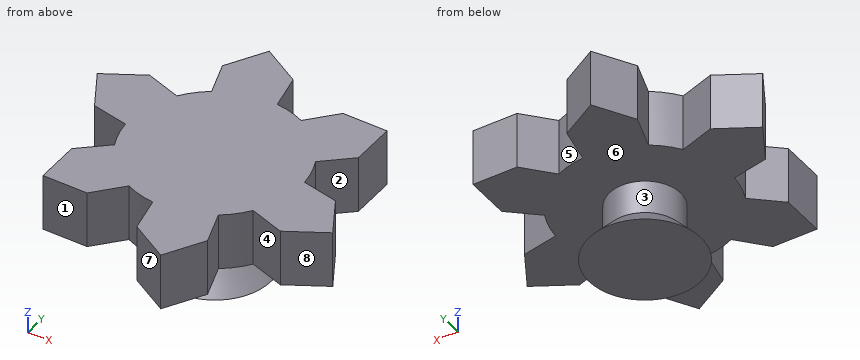
```python
from build123d import *

# Parameters (mm, degrees)
F1_DEPTH = 2.54
F2_R     = 1.5875
F3_DEPTH = 1.5
F4_R     = 2.5
F5_DEPTH = 1


with BuildPart() as f1:
    # F0 (on Top) → F1 (new body)
    with BuildSketch(Plane.XY):
        with BuildLine():
            ThreePointArc((1.6168332291, 3.4499203338), (1.7625208147, 3.3778129578), (1.905, 3.2995567884))
            ThreePointArc((1.905, 3.2995567884), (2.6940768363, 2.6940768363), (3.2995567884, 1.905))
            ThreePointArc((3.2995567884, 1.905), (3.3778129578, 1.7625208147), (3.4499203338, 1.6168332291))
            Line((3.4499203338, 1.6168332291), (4.669733183, 2.6960717102))
            Line((4.669733183, 2.6960717102), (4.669733183, 4.669733183))
            Line((4.669733183, 4.669733183), (2.6960717102, 4.669733183))
            Line((2.6960717102, 4.669733183), (1.6168332291, 3.4499203338))
        make_face()
        with BuildLine():
            Line((1.905, 3.2995567884), (0, 0))
            Line((0, 0), (3.2995567884, 1.905))
            ThreePointArc((3.2995567884, 1.905), (2.6940768363, 2.6940768363), (1.905, 3.2995567884))
        make_face()
        with BuildLine():
            ThreePointArc((0.3247415168, 3.7961352646), (0.1625186786, 3.806532238), (0, 3.81))
            Line((0, 3.81), (0, 0))
            Line((0, 0), (1.905, 3.2995567884))
            ThreePointArc((1.905, 3.2995567884), (1.7625208147, 3.3778129578), (1.6168332291, 3.4499203338))
            ThreePointArc((1.6168332291, 3.4499203338), (0.9861005618, 3.6801773982), (0.3247415168, 3.7961352646))
        make_face()
        with BuildLine():
            ThreePointArc((-1.905, 3.2995567884), (-0.9861005618, 3.6801773982), (0, 3.81))
            ThreePointArc((0, 3.81), (0.1625186786, 3.806532238), (0.3247415168, 3.7961352646))
            Line((0.3247415168, 3.7961352646), (0, 5.3921434204))
            Line((0, 5.3921434204), (-1.7092409739, 6.3789741568))
            Line((-1.7092409739, 6.3789741568), (-2.6960717102, 4.669733183))
            Line((-2.6960717102, 4.669733183), (-2.1793020355, 3.125178817))
            ThreePointArc((-2.1793020355, 3.125178817), (-2.0440114233, 3.2152942791), (-1.905, 3.2995567884))
        make_face()
        with BuildLine():
            Line((0, 0), (0, 3.81))
            ThreePointArc((0, 3.81), (-0.9861005618, 3.6801773982), (-1.905, 3.2995567884))
            Line((-1.905, 3.2995567884), (0, 0))
        make_face()
        with BuildLine():
            Line((-3.2995567884, 1.905), (0, 0))
            Line((0, 0), (-1.905, 3.2995567884))
            ThreePointArc((-1.905, 3.2995567884), (-2.0440114233, 3.2152942791), (-2.1793020355, 3.125178817))
            ThreePointArc((-2.1793020355, 3.125178817), (-2.6940768363, 2.6940768363), (-3.125178817, 2.1793020355))
            ThreePointArc((-3.125178817, 2.1793020355), (-3.2152942791, 2.0440114233), (-3.2995567884, 1.905))
        make_face()
        with BuildLine():
            ThreePointArc((-3.7961352646, -0.3247415168), (-3.806532238, -0.1625186786), (-3.81, 0))
            ThreePointArc((-3.81, 0), (-3.6801773982, 0.9861005618), (-3.2995567884, 1.905))
            ThreePointArc((-3.2995567884, 1.905), (-3.2152942791, 2.0440114233), (-3.125178817, 2.1793020355))
            Line((-3.125178817, 2.1793020355), (-4.669733183, 2.6960717102))
            Line((-4.669733183, 2.6960717102), (-6.3789741568, 1.7092409739))
            Line((-6.3789741568, 1.7092409739), (-5.3921434204, 0))
            Line((-5.3921434204, 0), (-3.7961352646, -0.3247415168))
        make_face()
        with BuildLine():
            Line((-3.81, 0), (0, 0))
            Line((0, 0), (-3.2995567884, 1.905))
            ThreePointArc((-3.2995567884, 1.905), (-3.6801773982, 0.9861005618), (-3.81, 0))
        make_face()
        with BuildLine():
            Line((-3.2995567884, -1.905), (0, 0))
            Line((0, 0), (-3.81, 0))
            ThreePointArc((-3.81, 0), (-3.806532238, -0.1625186786), (-3.7961352646, -0.3247415168))
            ThreePointArc((-3.7961352646, -0.3247415168), (-3.6801773982, -0.9861005618), (-3.4499203338, -1.6168332291))
            ThreePointArc((-3.4499203338, -1.6168332291), (-3.3778129578, -1.7625208147), (-3.2995567884, -1.905))
        make_face()
        with BuildLine():
            Line((-1.905, -3.2995567884), (0, 0))
            Line((0, 0), (-3.2995567884, -1.905))
            ThreePointArc((-3.2995567884, -1.905), (-2.6940768363, -2.6940768363), (-1.905, -3.2995567884))
        make_face()
        with BuildLine():
            ThreePointArc((-1.6168332291, -3.4499203338), (-1.7625208147, -3.3778129578), (-1.905, -3.2995567884))
            ThreePointArc((-1.905, -3.2995567884), (-2.6940768363, -2.6940768363), (-3.2995567884, -1.905))
            ThreePointArc((-3.2995567884, -1.905), (-3.3778129578, -1.7625208147), (-3.4499203338, -1.6168332291))
            Line((-3.4499203338, -1.6168332291), (-4.669733183, -2.6960717102))
            Line((-4.669733183, -2.6960717102), (-4.669733183, -4.669733183))
            Line((-4.669733183, -4.669733183), (-2.6960717102, -4.669733183))
            Line((-2.6960717102, -4.669733183), (-1.6168332291, -3.4499203338))
        make_face()
        with BuildLine():
            Line((0, -3.81), (0, 0))
            Line((0, 0), (-1.905, -3.2995567884))
            ThreePointArc((-1.905, -3.2995567884), (-1.7625208147, -3.3778129578), (-1.6168332291, -3.4499203338))
            ThreePointArc((-1.6168332291, -3.4499203338), (-0.9861005618, -3.6801773982), (-0.3247415168, -3.7961352646))
            ThreePointArc((-0.3247415168, -3.7961352646), (-0.1625186786, -3.806532238), (0, -3.81))
        make_face()
        with BuildLine():
            ThreePointArc((1.905, -3.2995567884), (0.9861005618, -3.6801773982), (0, -3.81))
            Line((0, -3.81), (0, -5.3921434204))
            Line((0, -5.3921434204), (1.7092409739, -6.3789741568))
            Line((1.7092409739, -6.3789741568), (2.6960717102, -4.669733183))
            Line((2.6960717102, -4.669733183), (2.1793020355, -3.125178817))
            ThreePointArc((2.1793020355, -3.125178817), (2.0440114233, -3.2152942791), (1.905, -3.2995567884))
        make_face()
        with BuildLine():
            Line((1.905, -3.2995567884), (0, 0))
            Line((0, 0), (0, -3.81))
            ThreePointArc((0, -3.81), (0.9861005618, -3.6801773982), (1.905, -3.2995567884))
        make_face()
        with BuildLine():
            Line((3.2995567884, -1.905), (0, 0))
            Line((0, 0), (1.905, -3.2995567884))
            ThreePointArc((1.905, -3.2995567884), (2.0440114233, -3.2152942791), (2.1793020355, -3.125178817))
            ThreePointArc((2.1793020355, -3.125178817), (2.6940768363, -2.6940768363), (3.125178817, -2.1793020355))
            ThreePointArc((3.125178817, -2.1793020355), (3.2152942791, -2.0440114233), (3.2995567884, -1.905))
        make_face()
        with BuildLine():
            Line((3.81, 0), (0, 0))
            Line((0, 0), (3.2995567884, -1.905))
            ThreePointArc((3.2995567884, -1.905), (3.6801773982, -0.9861005618), (3.81, 0))
        make_face()
        with BuildLine():
            Line((3.2995567884, 1.905), (0, 0))
            Line((0, 0), (3.81, 0))
            ThreePointArc((3.81, 0), (3.806532238, 0.1625186786), (3.7961352646, 0.3247415168))
            ThreePointArc((3.7961352646, 0.3247415168), (3.6801773982, 0.9861005618), (3.4499203338, 1.6168332291))
            ThreePointArc((3.4499203338, 1.6168332291), (3.3778129578, 1.7625208147), (3.2995567884, 1.905))
        make_face()
        with BuildLine():
            ThreePointArc((3.7961352646, 0.3247415168), (3.806532238, 0.1625186786), (3.81, 0))
            ThreePointArc((3.81, 0), (3.6801773982, -0.9861005618), (3.2995567884, -1.905))
            ThreePointArc((3.2995567884, -1.905), (3.2152942791, -2.0440114233), (3.125178817, -2.1793020355))
            Line((3.125178817, -2.1793020355), (4.669733183, -2.6960717102))
            Line((4.669733183, -2.6960717102), (6.3789741568, -1.7092409739))
            Line((6.3789741568, -1.7092409739), (5.3921434204, 0))
            Line((5.3921434204, 0), (3.7961352646, 0.3247415168))
        make_face()
        with BuildLine():
            Line((0, -5.3921434204), (0, -3.81))
            ThreePointArc((0, -3.81), (-0.1625186786, -3.806532238), (-0.3247415168, -3.7961352646))
            Line((-0.3247415168, -3.7961352646), (0, -5.3921434204))
        make_face()
    extrude(amount=F1_DEPTH)

    # F2 (on face) → F3 (join)
    with BuildSketch(Plane(origin=(0, 0, 0), x_dir=(1, 0, 0), z_dir=(0, 0, -1))):
        Circle(F2_R)
    extrude(amount=F3_DEPTH)

    # F4 (on face) → F5 (join)
    with BuildSketch(Plane(origin=(0, 0, -1.5), x_dir=(1, 0, 0), z_dir=(0, 0, -1))):
        Circle(F4_R)
    extrude(amount=F5_DEPTH)

    # F6 (on Right) → F7 (revolve, cut)
    with BuildSketch(Plane.YZ):
        Polygon((1.7, -1.5), (1.5990135726, -1.5), (2.5, -2.5), (2.5, -1.5), align=None)
    revolve(axis=Axis((0, 0, -2), (0, 0, 1)), mode=Mode.SUBTRACT)


solid = f1.part
```
Build history of the part. All positions in model axes, mm. Face numbers are marked on the shaded views. A direction names the side the tool comes from. Round coordinates to 2 decimals unless told otherwise and drop trailing zeros. Write each loop counter-clockwise with the first axis right and the second up, starting at its lowest first coordinate (ties: lowest second). Pieces come first, ordered by that corner, then holes. Notation, with made-up numbers: (42, 0.25) - (52, 0.25) arc R16 cw to (52, 11.25) - close; hole circle Ø3 at (77, -34.5). An arc over 180 degrees is marked (long way). Answer as CSV lines item,"result".
Q1. Tool access for the marked faces 1, 2, 3 and 4: list every direction of +Z, -Z, +X, -X, +Y, -Y with a clear straight run to the whole face (end or side of a thin tool).
Report:
face 1,"+Z, -Z, -X, -Y"
face 2,"+Z, -Z, +X"
face 3,"none"
face 4,"+Z, -Z, -Y"
Q2. Drill centre lines: probe 1 along Z at (x, y) = (-1.75, 5.5); probe 2 along Y at (x, z) = (0, -0.05); probe 3 along Y at (x, z) = (4, 0.45). Where is each one in solid material? Low to high. Write a range as [from, to].
Report:
probe 1,"z = [0, 2.54]"
probe 2,"y = [-1.59, 1.59]"
probe 3,"y = [-2.47, 0.28], [2.1, 4.67]"
Q3. Drop flat-ended pins along their axis: pin 1 (1.6 mm diameter, centred on x = -3.5, z = 1.5, fed in from -Y); pin 2 (2 mm diameter, centred on y = -3.5, z = 1.5, fed in from -X); pin 3 (4 mm diameter, centred on x = -1, y = -2.5, fed in from -Z); pin 4 (1.6 mm diameter, centred on x = 4, z = 2, fed in from +Y). Give the stop position or say it passes through.
Report:
pin 1,"stops at y = -4.67"
pin 2,"stops at x = -4.67"
pin 3,"stops at z = -2.5"
pin 4,"stops at y = 4.67"
Q4. Pull direction X, two halves, no side cores. Call the marked faces 5, 6, 7 and 8: +X half, -X half, draft (parallel to the pull), parting line (faces both ways), or undercut.
Report:
face 5,"undercut"
face 6,"draft"
face 7,"-X half"
face 8,"+X half"
Q5. Cut at B-B (z = -1.2). Write the cut outline in (x, y) (1 decimal).
Report:
outline,"circle Ø3.2 at (0, 0)"
